Check sheet for the modelled part. Datum: model origin and axes. Units: mm. Face numbers are marked on the shaded views. A direction names the side the tool comes from. Round coordinates to 2 decimals unless told otherwise and drop trailing zeros. Loops run counter-clockwise (first coordinate to the right, second up) from the corner with the lowest first, then second, coordinate; pieces in that order, holes last. Notation, with made-up numbers: (86.5, 47) - (122.5, 47) arc R5 cw to (122.5, 56) - close; hole circle Ø7 at (-23.5, -5). An arc over 180 degrees is marked (long way). Put each result on its own line as item: value.
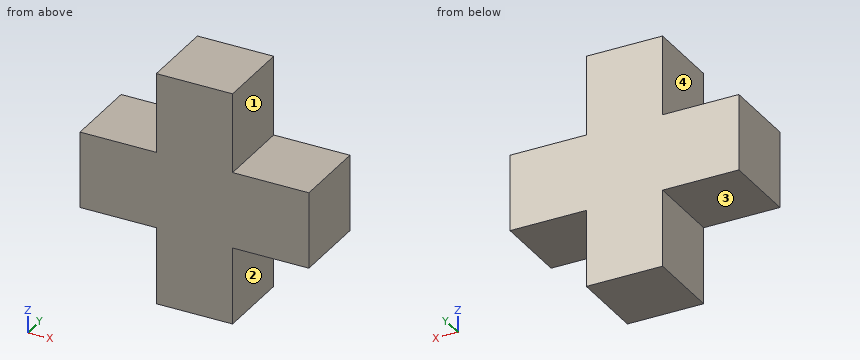
```python
from build123d import *

# Parameters (mm, degrees)
F0_W     = 19
F0_H     = 19
F1_DEPTH = 19


with BuildPart() as f1:
    # F0 (on Front) → F1 (new body)
    with BuildSketch(Plane.XZ):
        Polygon((7.165254, 19.838981), (-11.834746, 19.838981), (-11.834746, 0), (-11.834746, -19), (-11.834746, -38.161019), (-2.334746, -38.161019), (7.165254, -38.161019), (7.165254, -19), (7.165254, 0), align=None)
        with Locations((-21.334746, -9.5)):
            Rectangle(F0_W, F0_H)
        with Locations((16.665254, -9.5)):
            Rectangle(F0_W, F0_H)
    extrude(amount=F1_DEPTH)


solid = f1.part
```
Item 1: Section check B-B on z = -24.5. Enter the section's corners in (x, y), then the cut area to 3 significant figures.
Filled sheet:
outline: (-11.83, -19) - (7.17, -19) - (7.17, 0) - (-11.83, 0) - close
area: 361 mm²
Item 2: Tool access check on the marked faces 1, 2, 3 and 4. Record the directions out of +Z, -Z, +X, -X, +Y, -Y that give a thin tool (end or side, any length) a straight path to the whole face; none if there is none.
Filled sheet:
face 1: +Z, +X, +Y, -Y
face 2: -Z, +X, +Y, -Y
face 3: -Z, -X, +Y, -Y
face 4: +Z, -X, +Y, -Y
Item 3: Go/stop test with flat-tipped pins: pin 1 (5.5 mm diameter, centred on x = 18.5, y = -9, fed in from -Z); pin 2 (8 mm diameter, centred on y = -10, z = 14, fed in from -X); pin 3 (9.5 mm diameter, centred on y = -5, z = -27, fed in from +X). Record where each tip stops, or that it passes through.
Filled sheet:
pin 1: z = -19
pin 2: x = -11.83
pin 3: x = 7.17
Item 4: Section check A-A on y = -12.75. Enter the section's corners in (x, z), then the cut area to 3 significant figures.
Filled sheet:
outline: (-30.83, -19) - (-11.83, -19) - (-11.83, -38.16) - (7.17, -38.16) - (7.17, -19) - (26.17, -19) - (26.17, 0) - (7.17, 0) - (7.17, 19.84) - (-11.83, 19.84) - (-11.83, 0) - (-30.83, 0) - close
area: 1,820 mm²
Item 5: Thickness scan on line 1 (Z direction, x = -14.5, y = -14.5); line 2 (X direction, y = -13.5, z = 16.5). Record the ranges inside material, lowest first. Write a range as from..to.
Filled sheet:
line 1: -19..0
line 2: -11.83..7.17
Item 6: Section check C-C on x = 18.5. Enter the section's corners in (y, z).
Filled sheet:
outline: (-19, -19) - (0, -19) - (0, 0) - (-19, 0) - close
